For this review, take the finished solid that the model builds, in its own axes (mm). A direction names the side the tool comes from. Give positions to 0.01 mm unless a question says otherwise; leave off trailing zeros. Loops run counter-clockwise (first coordinate to the right, second up) from the corner with the lowest first, then second, coordinate; pieces in that order, holes last. Notation, with made-up numbers: (-16.75, -33.75) -> (23.25, -33.75) arc R32 ccw to (23.25, 0.25) -> close; hole circle Ø6 at (75, 19). An arc over 180 degrees is marked (long way). One line per question, with ' | ' between items. Start each with the question number.
(1) Consider section C-C (y = 11.9). Write out the cut boundary in (x, z).
(2) Wall thickness on probe 1 along Y at (x, z) = (4, 9.1); probe 2 along Y at (x, z) = (1.5, 6.5); probe 3 along X at (y, z) = (3.75, 5.5): over which ranges is each line inside the solid? List them lowest first.
(3) Draft analysis for pull direction Y (two halves, no side actions). For faces 4 (the flat face through (1.4, 8, 4)), 5 (the flat face through (6, 15.8, 5)), 6 (the flat face through (4, 12, 11.3)), state which applies: +Y half, -Y half, draft (parallel to the pull), parting line (faces both ways), or undercut.
(4) Consider section D-D (z = 10.25). Write out the cut boundary in (x, y).
(5) Consider section A-A (x = 4). Write out the cut boundary in (y, z), and give its area (3 significant figures).
(6) Tool access review of faces 1 (the cylindrical face through (6.217, 4.819, 10.387)), 2 (the flat face through (4, 4, 11.3)), 3 (the flat face through (10.08, 7.81, 5.24)): name each direction out of +Z, -Z, +X, -X, +Y, -Y from which nothing blocks a thin tool from reaching the whole face with its end or side.
(7) Consider section B-B (z = 1.75). Write out the cut boundary in (x, y).
(8) Insertion check: P1, Ø2, axis at x = 4, y = 12, coming from the -Z side; P2, Ø1, axis at y = 2.5, z = 3, coming from the +X side; P3, Ø4.5, axis at x = 4, y = 8, coming from the -Z side. Each pin has a flat end and moves straight along its axis. Give the tip position at first contact, or say it passes through.
Solid Edge part; units mm, degrees
sketch "Sketch1" plane through (0, 0, 0) normal (0, -1, 0) x (1, 0, 0)
  line L0 (0, 9.5) -> (8.55, 9.5)
  line L1 (16.25, 2.1) -> (8.55, 9.5)
  line L2 (16.25, 0) -> (16.25, 2.1)
  line L3 (0, 0) -> (16.25, 0)
  line L4 (0, 9.5) -> (0, 0)
extrude "Protrusion1" add sketch "Sketch1" against normal blind 15.8
sketch "Sketch2" plane through (8.125, 1.45, 4.75) normal (0, -1, 0) x (1, 0, 0)
  line L0 (6.175, -4.75) -> (6.175, -2.75)
  line L1 (6.175, -2.75) -> (5.175, -2.75)
  line L2 (-1.1815, 3.65) -> (5.175, -2.75)
  line L3 (-6.725, 3.65) -> (-1.1815, 3.65)
  line L4 (-6.725, 3.65) -> (-6.725, -4.75)
  line L5 (-6.725, -4.75) -> (6.175, -4.75)
extrude "ExtrudedCutout_1" cut sketch "Sketch2" against normal blind 12.9
sketch "Sketch3" plane through (4.275, 7.9, 9.5) normal (0, 0, 1) x (1, 0, 0)
  circle A0 centre (-0.275, 4) radius 2.4
  circle A1 centre (-0.275, -4) radius 2.4
extrude "ExtrudedProtrusion_2" add sketch "Sketch3" along normal blind 1.8
sketch "Sketch4" plane through (4.1717, 7.9, 8.4) normal (0, 0, -1) x (1, 0, 0)
  circle A0 centre (-0.1717, -4) radius 1.26
  circle A1 centre (-0.1717, 4) radius 1.26
extrude "Cutout1" cut sketch "Sketch4" against normal up to vertex (1.1 mm away)
A:
1) outline: (0, 0) -> (1.4, 0) -> (1.4, 8.4) -> (2.74, 8.4) -> (2.74, 9.5) -> (5.26, 9.5) -> (5.26, 8.4) -> (6.94, 8.4) -> (13.3, 2) -> (14.3, 2) -> (14.3, 0) -> (16.25, 0) -> (16.25, 2.1) -> (8.55, 9.5) -> (6.4, 9.5) -> (6.4, 11.3) -> (1.6, 11.3) -> (1.6, 9.5) -> (0, 9.5) -> close
2) probe 1: y = 0 to 2.64, 5.16 to 10.64, 13.16 to 15.8 | probe 2: y = 0 to 1.45, 14.35 to 15.8 | probe 3: x = 0 to 1.4, 9.82 to 12.71
3) face 4: undercut | face 5: +Y half | face 6: draft
4) outline: circle Ø4.8 at (4, 3.9); circle Ø4.8 at (4, 11.9)
5) outline: (0, 0) -> (1.45, 0) -> (1.45, 8.4) -> (2.64, 8.4) -> (2.64, 9.5) -> (5.16, 9.5) -> (5.16, 8.4) -> (10.64, 8.4) -> (10.64, 9.5) -> (13.16, 9.5) -> (13.16, 8.4) -> (14.35, 8.4) -> (14.35, 0) -> (15.8, 0) -> (15.8, 9.5) -> (14.3, 9.5) -> (14.3, 11.3) -> (9.5, 11.3) -> (9.5, 9.5) -> (6.3, 9.5) -> (6.3, 11.3) -> (1.5, 11.3) -> (1.5, 9.5) -> (0, 9.5) -> close | area: 53.5 mm^2
6) face 1: +Z | face 2: +Z, +X, -X, +Y, -Y | face 3: -Z
7) outline: (0, 0) -> (16.25, 0) -> (16.25, 15.8) -> (0, 15.8) -> close; hole (1.4, 1.45) -> (14.3, 1.45) -> (14.3, 14.35) -> (1.4, 14.35) -> close
8) P1: stops at z = 9.5 | P2: stops at x = 15.83 | P3: stops at z = 8.4
